Verification items for the finished model (mm, model axes). Face numbers are marked on the shaded views. A direction names the side the tool comes from. Round coordinates to 2 decimals unless told otherwise and drop trailing zeros. Order: outer loops, then holes, each group sorted by start corner. A loop starts at its lowest first (then second) coordinate and runs counter-clockwise, first axis right, second up. Notation, with made-up numbers: (-18, 10.25) -> (-14, 10.25) arc R17 ccw to (-14, 31.25) -> close; hole circle Ø3 at (70.25, 64.5). An arc over 180 degrees is marked (long way). Return JSON: item names as keys, results as strings. Group by question number.
1) Depth check by flat-ended pin: pin 1 (2.5 mm diameter, centred on x = 17.75, y = 38, fed in from +Z); pin 2 (3 mm diameter, centred on x = -16.5, y = 37.5, fed in from -Z); pin 3 (4 mm diameter, centred on x = -1.5, z = -2.5, fed in from +Y); pin 4 (6.5 mm diameter, centred on x = 18.5, y = 37.5, fed in from -Z). Enter the tip coordinate at first touch or a pass-through.
2) Section check B-B on z = -9. Enter the section's corners in (x, y), plus the area to 3 significant figures.
3) Section check D-D on x = 17.75. State how many separate pieces and enclosed holes the cut face has, plus the area to 3 significant figures.
4) Scan lines: L1, parallel to X at y = 7.4, z = -9; L2, parallel to Z at x = 17.75, y = 2.7; L3, parallel to Y at x = 17.75, z = 15.8. Record each from-to range of solid material in increasing order.
5) Section check C-C on y = 38. Enter the section's corners in (x, z), plus the area to 3 significant figures.
6) Tool access check on the marked faces 1 and 2. Record the directions out of +Z, -Z, +X, -X, +Y, -Y that give a thin tool (end or side, any length) a straight path to the whole face; none if there is none.
7) Section check A-A on z = 19. Enter the section's corners in (x, y).
```python
from build123d import *

# Parameters (mm, degrees)
SKETCH1_R              = 2
BASE_EXTRUSION_DEPTH   = 10
SKETCH2_R              = 3
FIRST_BASE_HOLES_DEPTH = 6
SKETCH5_W              = 45.5
SKETCH5_H              = 10
BOSS_EXTRUDE3_DEPTH    = 60
CUT_EXTRUDE2_REACH     = 72.011
SKETCH6_R              = 2
SKETCH7_R              = 3
CUT_EXTRUDE3_DEPTH     = 6


with BuildPart() as part:
    # Sketch1 → Base Extrusion (new body)
    with BuildSketch(Plane(origin=(0, 0, 0), x_dir=(1, 0, 0), z_dir=(0, 1, 0))):
        Polygon((-22.75, 14), (0, 14), (22.75, 14), (22.75, -14), (-22.75, -14), align=None)
        with Locations(Location((-17.75, 9, 0), (0, 0, 270))):
            Circle(SKETCH1_R, mode=Mode.SUBTRACT)
        with Locations(Location((-17.75, -9, 0), (0, 0, 270))):
            Circle(SKETCH1_R, mode=Mode.SUBTRACT)
        with Locations(Location((17.75, 9, 0), (0, 0, 270))):
            Circle(SKETCH1_R, mode=Mode.SUBTRACT)
        with Locations(Location((17.75, -9, 0), (0, 0, 270))):
            Circle(SKETCH1_R, mode=Mode.SUBTRACT)
    extrude(amount=BASE_EXTRUSION_DEPTH)

    # Sketch2 → First Base Holes (cut)
    with BuildSketch(Plane.XZ):
        with Locations(Location((-17.75, 9, 0), (0, 0, 270))):
            Circle(SKETCH2_R)
        with Locations(Location((-17.75, -9, 0), (0, 0, 270))):
            Circle(SKETCH2_R)
        with Locations(Location((17.75, -9, 0), (0, 0, 90))):
            Circle(SKETCH2_R)
        with Locations(Location((17.75, 9, 0), (0, 0, 90))):
            Circle(SKETCH2_R)
    extrude(amount=-FIRST_BASE_HOLES_DEPTH, mode=Mode.SUBTRACT)

    # Sketch5 → Boss-Extrude3 (add)
    with BuildSketch(Plane(origin=(0, 0, 0), x_dir=(1, 0, 0), z_dir=(0, 1, 0))):
        with Locations((0, -19)):
            Rectangle(SKETCH5_W, SKETCH5_H)
    extrude(amount=BOSS_EXTRUDE3_DEPTH)

    # Sketch6 → Cut-Extrude2 (cut, up to next)
    with BuildSketch(Plane(origin=(0, 0, 14), x_dir=(-1, 0, 0), z_dir=(0, 0, -1)), mode=Mode.PRIVATE) as cut_extrude2_sk1:
        with Locations((-17.75, 55)):
            Circle(SKETCH6_R)
    cut_extrude2_tool1 = extrude(cut_extrude2_sk1.sketch, amount=-CUT_EXTRUDE2_REACH, mode=Mode.PRIVATE) & part.part
    # Sketch6 → Cut-Extrude2 (cut, up to next)
    with BuildSketch(Plane(origin=(0, 0, 14), x_dir=(-1, 0, 0), z_dir=(0, 0, -1)), mode=Mode.PRIVATE) as cut_extrude2_sk2:
        with Locations((-17.75, 38)):
            Circle(SKETCH6_R)
    cut_extrude2_tool2 = extrude(cut_extrude2_sk2.sketch, amount=-CUT_EXTRUDE2_REACH, mode=Mode.PRIVATE) & part.part
    # Sketch6 → Cut-Extrude2 (cut, up to next)
    with BuildSketch(Plane(origin=(0, 0, 14), x_dir=(-1, 0, 0), z_dir=(0, 0, -1)), mode=Mode.PRIVATE) as cut_extrude2_sk3:
        with Locations((17.75, 55)):
            Circle(SKETCH6_R)
    cut_extrude2_tool3 = extrude(cut_extrude2_sk3.sketch, amount=-CUT_EXTRUDE2_REACH, mode=Mode.PRIVATE) & part.part
    # Sketch6 → Cut-Extrude2 (cut, up to next)
    with BuildSketch(Plane(origin=(0, 0, 14), x_dir=(-1, 0, 0), z_dir=(0, 0, -1)), mode=Mode.PRIVATE) as cut_extrude2_sk4:
        with Locations((17.75, 38)):
            Circle(SKETCH6_R)
    cut_extrude2_tool4 = extrude(cut_extrude2_sk4.sketch, amount=-CUT_EXTRUDE2_REACH, mode=Mode.PRIVATE) & part.part
    add(cut_extrude2_tool1.solids().sort_by_distance((17.75, 55, 14))[0], mode=Mode.SUBTRACT)
    add(cut_extrude2_tool2.solids().sort_by_distance((17.75, 38, 14))[0], mode=Mode.SUBTRACT)
    add(cut_extrude2_tool3.solids().sort_by_distance((-17.75, 55, 14))[0], mode=Mode.SUBTRACT)
    add(cut_extrude2_tool4.solids().sort_by_distance((-17.75, 38, 14))[0], mode=Mode.SUBTRACT)

    # Sketch7 → Cut-Extrude3 (cut)
    with BuildSketch(Plane(origin=(0, 0, 14), x_dir=(-1, 0, 0), z_dir=(0, 0, -1))):
        with Locations((-17.75, 55)):
            Circle(SKETCH7_R)
        with Locations((-17.75, 38)):
            Circle(SKETCH7_R)
        with Locations(Location((17.75, 38, 0), (0, 0, 180))):
            Circle(SKETCH7_R)
        with Locations(Location((17.75, 55, 0), (0, 0, 180))):
            Circle(SKETCH7_R)
    extrude(amount=-CUT_EXTRUDE3_DEPTH, mode=Mode.SUBTRACT)


solid = part.part
```
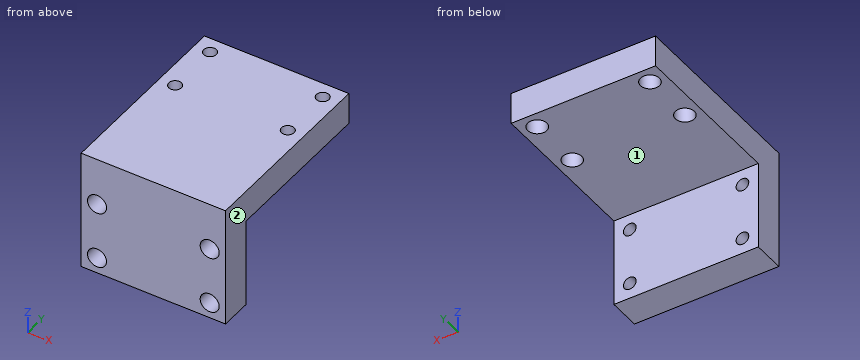
Check result:
{
 "1": {"pin 1": "through", "pin 2": "z = 20", "pin 3": "y = 10", "pin 4": "z = 14"},
 "2": {"outline": "(-22.75, 0) -> (-20.75, 0) -> (-20.75, 6) -> (-19.75, 6) -> (-19.75, 10) -> (-22.75, 10) -> close; (-15.75, 6) -> (-14.75, 6) -> (-14.75, 0) -> (14.75, 0) -> (14.75, 6) -> (15.75, 6) -> (15.75, 10) -> (-15.75, 10) -> close; (19.75, 6) -> (20.75, 6) -> (20.75, 0) -> (22.75, 0) -> (22.75, 10) -> (19.75, 10) -> close", "area": "351 mm^2"},
 "3": {"separate pieces": "5", "enclosed holes": "0", "area": "672 mm^2"},
 "4": {"L1": "-22.75 to -19.75, -15.75 to 15.75, 19.75 to 22.75", "L2": "-14 to -12, -6 to 6, 12 to 24", "L3": "0 to 35, 41 to 52, 58 to 60"},
 "5": {"outline": "(-22.75, 14) -> (-20.75, 14) -> (-20.75, 20) -> (-19.75, 20) -> (-19.75, 24) -> (-22.75, 24) -> close; (-15.75, 20) -> (-14.75, 20) -> (-14.75, 14) -> (14.75, 14) -> (14.75, 20) -> (15.75, 20) -> (15.75, 24) -> (-15.75, 24) -> close; (19.75, 20) -> (20.75, 20) -> (20.75, 14) -> (22.75, 14) -> (22.75, 24) -> (19.75, 24) -> close", "area": "351 mm^2"},
 "6": {"face 1": "-Z, +X, -X, +Y", "face 2": "+Z, -Z, +X, +Y, -Y"},
 "7": {"outline": "(-22.75, 0) -> (22.75, 0) -> (22.75, 60) -> (-22.75, 60) -> close; hole circle Ø6 at (-17.75, 38); hole circle Ø6 at (-17.75, 55); hole circle Ø6 at (17.75, 38); hole circle Ø6 at (17.75, 55)"}
}
